Work out the finished part from the listing and answer in its coordinate system (mm). Face numbers are marked on the shaded views. A direction names the side the tool comes from. Give positions to 0.01 mm unless a question says otherwise; leave off trailing zeros. One line per item, written item: value.
from build123d import *

# Parameters (mm, degrees)
SKETCH1_R                 = 16
BOSS_EXTRUDE1_DEPTH       = 43
SKETCH2_R                 = 12.5
BOSS_EXTRUDE2_DEPTH       = 58.4
SKETCH3_R                 = 9.5
BOSS_EXTRUDE3_DEPTH       = 2.25
SKETCH4_R                 = 5
BOSS_EXTRUDE4_DEPTH       = 2.6
SKETCH5_R                 = 3
CUT_EXTRUDE1_DEPTH        = 5
FILLET1_R                 = 1
M3X0_5_TAPPED_HOLE1_D     = 2.5
M3X0_5_TAPPED_HOLE1_DEPTH = 6.3
M3X0_5_TAPPED_HOLE1_TIP   = 0.751075774


with BuildPart() as part:
    # Sketch1 → Boss-Extrude1 (new body)
    with BuildSketch(Plane.XY):
        Circle(SKETCH1_R)
    extrude(amount=BOSS_EXTRUDE1_DEPTH)

    # Sketch2 → Boss-Extrude2 (add)
    with BuildSketch(Plane.XY.offset(43)):
        Circle(SKETCH2_R)
    extrude(amount=BOSS_EXTRUDE2_DEPTH)

    # Sketch3 → Boss-Extrude3 (add)
    with BuildSketch(Plane(origin=(0, 0, 0), x_dir=(-1, 0, 0), z_dir=(0, 0, -1))):
        Circle(SKETCH3_R)
    extrude(amount=BOSS_EXTRUDE3_DEPTH)

    # Sketch4 → Boss-Extrude4 (add)
    with BuildSketch(Plane(origin=(0, 0, -2.25), x_dir=(-1, 0, 0), z_dir=(0, 0, -1))):
        Circle(SKETCH4_R)
    extrude(amount=BOSS_EXTRUDE4_DEPTH)

    # Sketch5 → Cut-Extrude1 (cut)
    with BuildSketch(Plane(origin=(0, 0, -4.85), x_dir=(-1, 0, 0), z_dir=(0, 0, -1))):
        Circle(SKETCH5_R)
    extrude(amount=-CUT_EXTRUDE1_DEPTH, mode=Mode.SUBTRACT)

    # Fillet1
    fillet1_edges = [part.edges().sort_by_distance(p)[0] for p in [
        (-16, 0, 43),
        (-12.5, 0, 43),
        (-12.5, 0, 101.4),
    ]]
    fillet(fillet1_edges, radius=FILLET1_R)

    # M3x0.5 Tapped Hole1
    with Locations(Plane(origin=(0, 0, 0), x_dir=(-1, 0, 0), z_dir=(0, 0, -1))):
        with Locations((0, 13), (-13, 0), (0, -13), (13, 0)):
            Hole(M3X0_5_TAPPED_HOLE1_D / 2, depth=M3X0_5_TAPPED_HOLE1_DEPTH)
            with Locations((0, 0, -(M3X0_5_TAPPED_HOLE1_DEPTH + M3X0_5_TAPPED_HOLE1_TIP / 2))):  # 118° drill point
                Cone(0, M3X0_5_TAPPED_HOLE1_D / 2, M3X0_5_TAPPED_HOLE1_TIP, mode=Mode.SUBTRACT)


solid = part.part
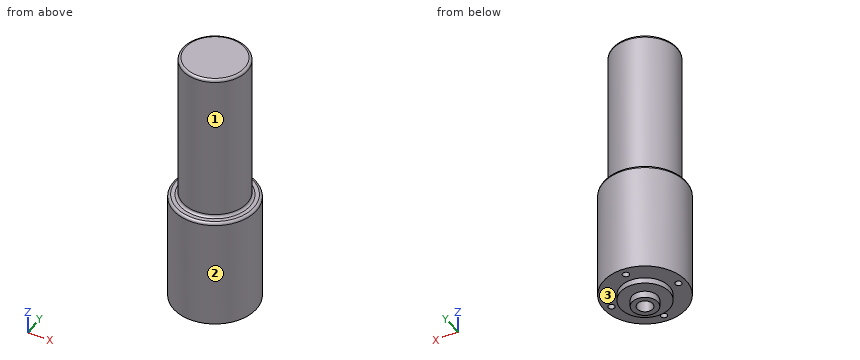
1. Flat-ended cylindrical pins translate along their axes: pin 1 Ø3 at (x, z) = (-1.5, 61.5) entering from -Y; pin 2 Ø2 at (x, y) = (13, 0) entering from -Z; pin 3 Ø6 at (x, y) = (4, 11.5) entering from -Z; pin 4 Ø5 at (y, z) = (2.5, 32) entering from +X. Find the tip coordinate at first contact, or state that the pin passes through.
Output:
pin 1: stops at y = -12.5
pin 2: stops at z = 6.45
pin 3: stops at z = -2.25
pin 4: stops at x = 16
2. Find the intervals of material crossed by line 1 along Z through (x, y) = (13, -7); line 2 along Y through (x, z) = (-5.5, 0.5); line 3 along X through (y, z) = (13, 1.75), in increasing order.
Output:
line 1: z = 0 to 43
line 2: y = -15.02 to 15.02
line 3: x = -9.33 to -1.25, 1.25 to 9.33
3. For the marked faces 1, 2 and 3, determine the directions among +Z, -Z, +X, -X, +Y, -Y from which every point of the face is accessible in a straight line to the end or side of a thin tool.
Output:
face 1: +Z
face 2: +Z, -Z
face 3: -Z
